Here's how the part is built. I have some questions about the finished solid (model axes, mm). Round coordinates to 2 decimals unless told otherwise and drop trailing zeros. Loops run counter-clockwise (first coordinate to the right, second up) from the corner with the lowest first, then second, coordinate; pieces in that order, holes last. Notation, with made-up numbers: (79.5, -13) -> (113.5, -13) arc R31 ccw to (113.5, 11) -> close; hole circle Ø10 at (-5, -8.75). An arc over 180 degrees is marked (long way). One line per item, written item: value. Start each with the question number.
```python
from build123d import *

# Parameters (mm, degrees)
F0_R     = 12.5
F1_DEPTH = 7.5
F1_TAPER = 60
F3_T     = -0.8
F2_R     = 1
F4_DEPTH = 25


with BuildPart() as f1:
    # F0 (on Top) → F1 (new body)
    with BuildSketch(Plane.XY):
        Circle(F0_R)
    extrude(amount=F1_DEPTH, taper=F1_TAPER)

    # F3
    f3_openings = [f1.faces().sort_by_distance(p)[0] for p in [
        (0, 0, 0),
    ]]
    offset(amount=F3_T, openings=f3_openings)

    # F2 (on Top) → F4 (cut)
    with BuildSketch(Plane.XY):
        Circle(F2_R)
    extrude(amount=F4_DEPTH, mode=Mode.SUBTRACT)


solid = f1.part
```
Q1. If I drill on line 1 along X through (y, z) = (0, 6.1); line 2 along X through (y, z) = (-3, 3.75), over which ranges is the centre line in solid material (lowest first)?
Q2. I want a section at A-A on x = 0. Please give me the cut outline in (y, z).
Q3. If we mould it in two halves opening along Y, with no side actions, what happens to faces 1 (the cylindrical face through (0, -1, 6)), 2 (the conical face through (-1.237, -0.948, 6.317)), 3 (the flat face through (0.9, 11.2, 0)), 4 (the conical face through (-0.321, -1.445, 5.438))? For each: released by +Y, released by -Y, zero draft, split by the parting line, or undercut.
Q4. I want a section at C-C on z = 4.5. Please give me the cut outline in (x, y), plus the area to 3 significant figures.
Q5. I want a section at D-D on z = 2. Please give me the cut outline in (x, y), plus the area to 3 significant figures.
Q6. Will these pins go through, and if not, where does the flat tip stop? P1, Ø1, axis at x = 5.5, z = 5.5, coming from the +Y side; P2, Ø4, axis at x = 2.5, y = 7.5, coming from the +Z side.
Answers below:
1. line 1: x = -1.93 to -1, 1 to 1.93
1. line 2: x = -5.2 to -3.23, 3.23 to 5.2
2. outline: (-12.5, 0) -> (-10.9, 0) -> (-1, 5.72) -> (-1, 6.64) -> close; (1, 5.72) -> (10.9, 0) -> (12.5, 0) -> (1, 6.64) -> close
3. face 1: undercut
3. face 2: split by the parting line
3. face 3: zero draft
3. face 4: undercut
4. outline: circle Ø9.41 at (0, 0); hole circle Ø6.21 at (0, 0)
4. area: 39.3 mm^2
5. outline: circle Ø18.07 at (0, 0); hole circle Ø14.87 at (0, 0)
5. area: 82.8 mm^2
6. P1: passes through
6. P2: stops at z = 3.81
